Design review of the part built by this model. Coordinates are the model's own, in mm. A direction names the side the tool comes from. Give positions to 0.01 mm unless a question says otherwise; leave off trailing zeros. Loops run counter-clockwise (first coordinate to the right, second up) from the corner with the lowest first, then second, coordinate; pieces in that order, holes last. Notation, with made-up numbers: (-7.5, -4.75) -> (37.5, -4.75) arc R28 ccw to (37.5, 15.25) -> close; hole circle Ø5 at (40, -6.75). An arc over 180 degrees is marked (long way). Use a Markdown table: item, result. Add a question column.
1. Add section C-C (x = 1.3). Count the separate pieces of the cut face and the enclosed holes in it, and give its area (3 significant figures).
2. Add section B-B (z = 39.5). State the section outline as (x, y) points.
3. For pin 1 Ø1.5 at (x, y) = (2, 0) entering from +Z, flat-tipped, find the tip position at first contact; note if it passes through.
4. For faces 1 (the flat face through (1, 0, -5.55)), 2 (the flat face through (2, -9.1, -14)), list the 3-axis set-ups (+Z, -Z, +X, -X, +Y, -Y) from which the entire face can be reached by the end or side of a thin tool; tool diameter is ignored.
5. To check wall thickness, follow line 1 (Z direction, x = 1.8, y = 2.5); line 2 (Y direction, x = 1, z = -63.5); line 3 (Y direction, x = 0.8, z = -47.5). State the ranges of each line that lie inside material, in increasing order.
6. Add section A-A (y = -1.5). State the section outline as (x, z) points, and give its area (3 significant figures).
```python
from build123d import *

# Parameters (mm, degrees)
SKETCH_1_W      = 36.4
SKETCH_1_H      = 11.2
EXTRUDE_1_DEPTH = 3
SKETCH_2_W      = 22.91
SKETCH_2_H      = 11.2
EXTRUDE_2_DEPTH = 3


with BuildPart() as part:
    # 草图1 → 凸台-拉伸1 (new body)
    with BuildSketch(Plane(origin=(0, 0, 0), x_dir=(0, 0, -1), z_dir=(1, 0, 0))):
        with BuildLine():
            ThreePointArc((-44.9, -4.05), (-45.20753788, -4.79246212), (-45.95, -5.1))
            Line((-45.95, -5.1), (-49.05, -5.1))
            Line((-49.05, -5.1), (-49.05, -9.1))
            Line((-49.05, -9.1), (49.05, -9.1))
            Line((49.05, -9.1), (49.05, -5.1))
            Line((49.05, -5.1), (45.95, -5.1))
            ThreePointArc((45.95, -5.1), (44.9, -4.05), (45.95, -3))
            Line((45.95, -3), (45.95, 3))
            ThreePointArc((45.95, 3), (44.9, 4.05), (45.95, 5.1))
            Line((45.95, 5.1), (49.05, 5.1))
            Line((49.05, 5.1), (49.05, 9.1))
            Line((49.05, 9.1), (-49.05, 9.1))
            Line((-49.05, 9.1), (-49.05, 5.1))
            Line((-49.05, 5.1), (-45.95, 5.1))
            ThreePointArc((-45.95, 5.1), (-45.20753788, 4.79246212), (-44.9, 4.05))
            ThreePointArc((-44.9, 4.05), (-45.20753788, 3.30753788), (-45.95, 3))
            Line((-45.95, 3), (-45.95, -3))
            ThreePointArc((-45.95, -3), (-45.20753788, -3.30753788), (-44.9, -4.05))
        make_face()
        with Locations((-23.75, 0)):
            Rectangle(SKETCH_1_W, SKETCH_1_H, mode=Mode.SUBTRACT)
        with BuildLine():
            ThreePointArc((2.6, -4.05), (2.29246212, -4.79246212), (1.55, -5.1))
            Line((1.55, -5.1), (-1.55, -5.1))
            ThreePointArc((-1.55, -5.1), (-2.6, -4.05), (-1.55, -3))
            Line((-1.55, -3), (-1.55, 3))
            ThreePointArc((-1.55, 3), (-2.6, 4.05), (-1.55, 5.1))
            Line((-1.55, 5.1), (1.55, 5.1))
            ThreePointArc((1.55, 5.1), (2.29246212, 4.79246212), (2.6, 4.05))
            ThreePointArc((2.6, 4.05), (2.29246212, 3.30753788), (1.55, 3))
            Line((1.55, 3), (1.55, -3))
            ThreePointArc((1.55, -3), (2.29246212, -3.30753788), (2.6, -4.05))
        make_face(mode=Mode.SUBTRACT)
        with Locations((23.75, 0)):
            Rectangle(SKETCH_1_W, SKETCH_1_H, mode=Mode.SUBTRACT)
    extrude(amount=EXTRUDE_1_DEPTH)

    # 草图2 → 凸台-拉伸2 (add)
    with BuildSketch(Plane(origin=(3, 0, 0), x_dir=(0, 0, -1), z_dir=(1, 0, 0))):
        with BuildLine():
            Line((49.05, -5.1), (49.05, -9.1))
            Line((49.05, -9.1), (78.96, -9.1))
            Line((78.96, -9.1), (78.96, 9.1))
            Line((78.96, 9.1), (49.05, 9.1))
            Line((49.05, 9.1), (49.05, 5.1))
            ThreePointArc((49.05, 5.1), (49.79246212, 4.79246212), (50.1, 4.05))
            ThreePointArc((50.1, 4.05), (49.79246212, 3.30753788), (49.05, 3))
            Line((49.05, 3), (49.05, -3))
            ThreePointArc((49.05, -3), (49.79246212, -3.30753788), (50.1, -4.05))
            ThreePointArc((50.1, -4.05), (49.79246212, -4.79246212), (49.05, -5.1))
        make_face()
        with Locations((64.505, 0)):
            Rectangle(SKETCH_2_W, SKETCH_2_H, mode=Mode.SUBTRACT)
    extrude(amount=-EXTRUDE_2_DEPTH)


solid = part.part
```
Taken from the geometry:
| question | item | result |
|---|---|---|
| 1 | separate pieces | 1 |
| 1 | enclosed holes | 5 |
| 1 | area | 1,150 mm^2 |
| 2 | outline | (0, -9.1) -> (3, -9.1) -> (3, -5.6) -> (0, -5.6) -> close; (0, 5.6) -> (3, 5.6) -> (3, 9.1) -> (0, 9.1) -> close |
| 3 | pin 1 | stops at z = 45.95 |
| 4 | face 1 | +X, -X |
| 4 | face 2 | +Z, -Z, +X, -X, -Y |
| 5 | line 1 | z = -78.96 to -75.96, -53.05 to -49.05, -45.95 to -41.95, -5.55 to -1.55, 1.55 to 5.55, 41.95 to 45.95 |
| 5 | line 2 | y = -9.1 to -5.6, 5.6 to 9.1 |
| 5 | line 3 | y = -9.1 to -5.1, 5.1 to 9.1 |
| 6 | outline | (0, -78.96) -> (3, -78.96) -> (3, -75.96) -> (0, -75.96) -> close; (0, -53.05) -> (3, -53.05) -> (3, -49.05) -> (0, -49.05) -> close; (0, -45.95) -> (3, -45.95) -> (3, -41.95) -> (0, -41.95) -> close; (0, -5.55) -> (3, -5.55) -> (3, -1.55) -> (0, -1.55) -> close; (0, 1.55) -> (3, 1.55) -> (3, 5.55) -> (0, 5.55) -> close; (0, 41.95) -> (3, 41.95) -> (3, 45.95) -> (0, 45.95) -> close |
| 6 | area | 69.0 mm^2 |
